The listing builds one solid part. Answer for the finished solid, in the listing's coordinates (mm). A direction names the side the tool comes from. Round coordinates to 2 decimals unless told otherwise and drop trailing zeros. Use a Markdown table: item, result. Add a question column.
1) Find the intervals of material crossed by probe 1 along Y at (x, z) = (0, 6.25) (3 decimals); probe 2 along Y at (x, z) = (0, 17.45); probe 3 along Y at (x, z) = (33.5, 12.75), in increasing order. Write a range as from..to.
2) Determine the mould class of faces 4 (the cylindrical face through (36.172, -32.648, 11.997)), 5 (the flat face through (-1, 19, 0)), 6 (the cylindrical face through (42.54, 42.64, 9.66)), 7 (the flat face through (-1, -44.45, 12)) for opening direction Y: +Y half, -Y half, draft (parallel to the pull), parting line (faces both ways), or undercut.
3) Each of these flat-tipped pins is pushed along its axis until it touches: P1, Ø17.5, axis at x = 0, y = -32.5, coming from the -Z side; P2, Ø6, axis at x = -34.8, y = -34.8, coming from the +Z side; P3, Ø2.5, axis at x = -14, z = 2, coming from the -Y side. Where does it stop, or does it pass through?
4) A tool of negligible diameter and unlimited length cuts with its end or side. For faces 1 (the flat face through (44.45, -1, 9)), 2 (the flat face through (-1, -22.86, 2)), 3 (the cylindrical face through (34.824, 10.967, 17.798)), from which of +Z, -Z, +X, -X, +Y, -Y can it reach the whole face along a straight path? Write none if from no direction.
5) A cutting plane is placed at A-A (y = 0). State how many separate pieces and enclosed holes the cut face has, then the cut area to 3 significant figures.
```python
from build123d import *

# Parameters (mm, degrees)
SKETCH1_W                                     = 88.9
SKETCH1_H                                     = 88.9
BOSS_EXTRUDE1_DEPTH                           = 19.05
SKETCH2_R                                     = 36.51
CUT_EXTRUDE1_DEPTH                            = 2.54
SKETCH5_R                                     = 15.875
CUT_EXTRUDE3_DEPTH                            = 65.993731236
SKETCH4_W                                     = 4.7625
SKETCH4_H                                     = 21.59
CUT_EXTRUDE2_DEPTH                            = 102.202346811
FILLET1_R                                     = 6.35
CBORE_FOR_1_4_SOCKET_HEAD_CAP_SCREW1_AT_COUNT = 2
CBORE_FOR_1_4_SOCKET_HEAD_CAP_SCREW1_AT_PITCH = 57.15


# Read off the part's stored shape, not the designer's step: 1/4-20 Tapped Hole2
with BuildPart() as part:
    # Sketch1 → Boss-Extrude1 (new body)
    with BuildSketch(Plane.XY):
        Rectangle(SKETCH1_W, SKETCH1_H)
    extrude(amount=BOSS_EXTRUDE1_DEPTH)

    # Sketch2 → Cut-Extrude1 (cut)
    with BuildSketch(Plane.XY.offset(19.05)):
        Circle(SKETCH2_R)
    extrude(amount=-CUT_EXTRUDE1_DEPTH, mode=Mode.SUBTRACT)

    # Sketch5 → Cut-Extrude3 (cut, through all)
    with BuildSketch(Plane.XY.offset(16.51)):
        Circle(SKETCH5_R)
    extrude(amount=-CUT_EXTRUDE3_DEPTH, mode=Mode.SUBTRACT)

    # Sketch4 → Cut-Extrude2 (cut, through all)
    with BuildSketch(Plane.ZY.offset(44.45)):
        with Locations((2.38125, -33.655)):
            Rectangle(SKETCH4_W, SKETCH4_H)
    extrude(amount=-CUT_EXTRUDE2_DEPTH, mode=Mode.SUBTRACT)

    # Fillet1
    fillet1_edges = [part.edges().sort_by_distance(p)[0] for p in [
        (44.45, -44.45, 11.90625),
        (-44.45, -44.45, 11.90625),
        (-44.45, 44.45, 9.525),
        (44.45, 44.45, 9.525),
    ]]
    fillet(fillet1_edges, radius=FILLET1_R)

    # 1/4-20 Tapped Hole2 outline → 1/4-20 Tapped Hole2 (revolve, cut)
    with BuildSketch(Plane(origin=(34.8, 34.8, 0), x_dir=(1, 0, 0), z_dir=(0, -1, 0))):
        Polygon((0, 0), (3.1877, 0), (2.5527, 0.635), (2.5527, 18.415), (3.1877, 19.05), (0, 19.05), align=None)
    revolve(axis=Axis((34.8, 34.8, 0), (0, 0, 1)), mode=Mode.SUBTRACT)

    # 1_4-20 Tapped Hole2 2 outline → 1_4-20 Tapped Hole2 2 (revolve, cut)
    with BuildSketch(Plane(origin=(-34.8, -34.8, 0), x_dir=(1, 0, 0), z_dir=(0, -1, 0))):
        Polygon((0, 4.7625), (3.1877, 4.7625), (2.5527, 5.3975), (2.5527, 18.415), (3.1877, 19.05), (0, 19.05), align=None)
    revolve(axis=Axis((-34.8, -34.8, 0), (0, 0, 1)), mode=Mode.SUBTRACT)

    # 1_4-20 Tapped Hole2 3 outline → 1_4-20 Tapped Hole2 3 (revolve, cut)
    with BuildSketch(Plane(origin=(-34.8, 34.8, 0), x_dir=(1, 0, 0), z_dir=(0, -1, 0))):
        Polygon((0, 0), (3.1877, 0), (2.5527, 0.635), (2.5527, 18.415), (3.1877, 19.05), (0, 19.05), align=None)
    revolve(axis=Axis((-34.8, 34.8, 0), (0, 0, 1)), mode=Mode.SUBTRACT)

    # 1_4-20 Tapped Hole2 4 outline → 1_4-20 Tapped Hole2 4 (revolve, cut)
    with BuildSketch(Plane(origin=(34.8, -34.8, 0), x_dir=(1, 0, 0), z_dir=(0, -1, 0))):
        Polygon((0, 4.7625), (3.1877, 4.7625), (2.5527, 5.3975), (2.5527, 18.415), (3.1877, 19.05), (0, 19.05), align=None)
    revolve(axis=Axis((34.8, -34.8, 0), (0, 0, 1)), mode=Mode.SUBTRACT)

    # Sketch9 → CBORE for 1/4 Socket Head Cap Screw1 (revolve, cut)
    with BuildSketch(Plane(origin=(28.575, 0, 19.05), x_dir=(0, -1, 0), z_dir=(1, 0, 0))):
        Polygon((0, 0), (0, 19.05), (4.0132, 19.05), (3.3782, 18.415), (3.3782, 7.62), (5.55625, 7.62), (5.55625, 0.635), (6.19125, 0), align=None)
    cbore_for_1_4_socket_head_cap_screw1 = revolve(axis=Axis((28.575, 0, 25.4), (0, 0, -1)), mode=Mode.SUBTRACT)

    # CBORE for 1/4 Socket Head Cap Screw1 at: CBORE for 1/4 Socket Head Cap Screw1 ×2
    with Locations(*[(-i * CBORE_FOR_1_4_SOCKET_HEAD_CAP_SCREW1_AT_PITCH, 0, 0) for i in range(1, CBORE_FOR_1_4_SOCKET_HEAD_CAP_SCREW1_AT_COUNT)]):
        add(cbore_for_1_4_socket_head_cap_screw1, mode=Mode.SUBTRACT)


solid = part.part
```
Entries:
| question | item | result |
|---|---|---|
| 1 | probe 1 | y = -44.45..-15.875, 15.875..44.45 |
| 1 | probe 2 | y = -44.45..-36.51, 36.51..44.45 |
| 1 | probe 3 | y = -44.45..-37, -32.6..-2.57, 2.57..32.6, 37..44.45 |
| 2 | face 4 | undercut |
| 2 | face 5 | draft |
| 2 | face 6 | +Y half |
| 2 | face 7 | -Y half |
| 3 | P1 | stops at z = 4.76 |
| 3 | P2 | stops at z = 18.86 |
| 3 | P3 | stops at y = -22.86 |
| 4 | face 1 | +Z, -Z, +X, +Y, -Y |
| 4 | face 2 | -Z, +X, -X, -Y |
| 4 | face 3 | +Z |
| 5 | separate pieces | 4 |
| 5 | enclosed holes | 0 |
| 5 | area | 716 mm² |
